```python
from build123d import *

# Parameters (mm, degrees)
BOSS_EXTRUDE1_DEPTH = 0.5
FILLET1_R           = 0.5
FILLET2_R           = 0.1
CUT_EXTRUDE1_REACH  = 9.579
SKETCH2_R           = 0.25


with BuildPart() as part:
    # Sketch1 → Boss-Extrude1 (new body)
    with BuildSketch(Plane.XY):
        with BuildLine():
            Line((-3.674234614, 0.75), (-5.674234614, 0.75))
            Line((-5.674234614, 0.75), (-5.674234614, 1.75))
            Line((-5.674234614, 1.75), (-4.333748499, 1.75))
            ThreePointArc((-4.333748499, 1.75), (5.35, 0), (-4.333748499, -1.75))
            Line((-4.333748499, -1.75), (-5.674234614, -1.75))
            Line((-5.674234614, -1.75), (-5.674234614, -0.75))
            Line((-5.674234614, -0.75), (-3.674234614, -0.75))
            ThreePointArc((-3.674234614, -0.75), (3.75, 0), (-3.674234614, 0.75))
        make_face()
    extrude(amount=BOSS_EXTRUDE1_DEPTH)

    # Fillet1
    fillet1_edges = [part.edges().sort_by_distance(p)[0] for p in [
        (-5.674234614, 1.75, 0.25),
        (-4.333748499, 1.75, 0.25),
        (-4.333748499, -1.75, 0.25),
        (-5.674234614, -1.75, 0.25),
        (-3.674234614, -0.75, 0.25),
        (-3.674234614, 0.75, 0.25),
    ]]
    fillet(fillet1_edges, radius=FILLET1_R)

    # Fillet2
    fillet2_edges = [part.edges().sort_by_distance(p)[0] for p in [
        (-5.674234614, -0.75, 0.25),
        (-5.674234614, 0.75, 0.25),
    ]]
    fillet(fillet2_edges, radius=FILLET2_R)

    # Sketch2 → Cut-Extrude1 (cut, up to next)
    with BuildSketch(Plane.XY.offset(0.5), mode=Mode.PRIVATE) as cut_extrude1_sk1:
        with Locations((-5.124234614, 1.3)):
            Circle(SKETCH2_R)
    cut_extrude1_tool1 = extrude(cut_extrude1_sk1.sketch, amount=-CUT_EXTRUDE1_REACH, mode=Mode.PRIVATE) & part.part
    # Sketch2 → Cut-Extrude1 (cut, up to next)
    with BuildSketch(Plane.XY.offset(0.5), mode=Mode.PRIVATE) as cut_extrude1_sk2:
        with Locations((-5.124234614, -1.3)):
            Circle(SKETCH2_R)
    cut_extrude1_tool2 = extrude(cut_extrude1_sk2.sketch, amount=-CUT_EXTRUDE1_REACH, mode=Mode.PRIVATE) & part.part
    add(cut_extrude1_tool1.solids().sort_by_distance((-5.124235, 1.3, 0.5))[0], mode=Mode.SUBTRACT)
    add(cut_extrude1_tool2.solids().sort_by_distance((-5.124235, -1.3, 0.5))[0], mode=Mode.SUBTRACT)


solid = part.part
```
Model file for the job. Use its own axes, mm. Give positions to 0.01 mm unless a question says otherwise; leave off trailing zeros. Loops run counter-clockwise (first coordinate to the right, second up) from the corner with the lowest first, then second, coordinate; pieces in that order, holes last. Notation, with made-up numbers: (-12, 29) -> (-8, 29) arc R22 ccw to (-8, 48) -> close; hole circle Ø11 at (17, 78.25). An arc over 180 degrees is marked (long way). Use CSV: the item, a comma, the result in double quotes. Start each with the question number.
1) Slice it at A-A on y = 3. Give the cut face in (x, z).
2) Wall check: line 1 (Y direction, x = 0, z = 0.2); line 2 (Y direction, x = -3, z = 0.3); line 3 (Y direction, x = -5, z = 0.4). Give the ranges that are in metal, low to high.
3) Mould opens along X. For faces 1 (the flat face through (4, 2, 0)), 2 (the cylindrical face through (3.747, -0.149, 0.246)), 3 (the cylindrical face through (5.346, 0.19, 0.246)) say: released by +X, released by -X, zero draft, split by the parting line, or undercut.
4) Slice it at C-C on z = 0.25. Give the cut face in (x, y).
5) Slice it at D-D on y = 0. Give the cut face in (x, z).
6) Slice it at B-B on x = 0.35. Give the cut face in (y, z), plus the area to 3 significant figures.
Computed values:
1,outline,"(-3.65, 0) -> (-2.25, 0) -> (-2.25, 0.5) -> (-3.65, 0.5) -> close; (2.25, 0) -> (4.35, 0) -> (4.35, 0.5) -> (2.25, 0.5) -> close"
2,line 1,"y = -4.99 to -3.75, 3.75 to 4.99"
2,line 2,"y = -3.71 to -2.25, 2.25 to 3.71"
2,line 3,"y = -1.75 to -1.52, -1.08 to -0.75, 0.75 to 1.08, 1.52 to 1.75"
3,face 1,"zero draft"
3,face 2,"undercut"
3,face 3,"split by the parting line"
4,outline,"(-5.67, -1.25) arc R0.5 ccw to (-5.17, -1.75) -> (-4.67, -1.75) arc R0.5 cw to (-4.21, -2.05) arc R5 ccw (long way) to (-4.21, 2.05) arc R0.5 cw to (-4.67, 1.75) -> (-5.17, 1.75) arc R0.5 ccw to (-5.67, 1.25) -> (-5.67, 0.85) arc R0.1 ccw to (-5.57, 0.75) -> (-4.06, 0.75) arc R0.5 ccw to (-3.58, 1.1) arc R3.75 cw (long way) to (-3.58, -1.1) arc R0.5 ccw to (-4.06, -0.75) -> (-5.57, -0.75) arc R0.1 ccw to (-5.67, -0.85) -> close; hole circle Ø0.5 at (-5.12, -1.3); hole circle Ø0.5 at (-5.12, 1.3)"
5,outline,"(3.75, 0) -> (5.35, 0) -> (5.35, 0.5) -> (3.75, 0.5) -> close"
6,outline,"(-5, 0) -> (-3.73, 0) -> (-3.73, 0.5) -> (-5, 0.5) -> close; (3.73, 0) -> (5, 0) -> (5, 0.5) -> (3.73, 0.5) -> close"
6,area,"1.27 mm^2"
